Here's how the part is built. I have some questions about the finished solid (model axes, mm). Round coordinates to 2 decimals unless told otherwise and drop trailing zeros. Loops run counter-clockwise (first coordinate to the right, second up) from the corner with the lowest first, then second, coordinate; pieces in that order, holes last. Notation, with made-up numbers: M 46,22.5 L 58,22.5 A17 cw 58,50.5 Z; hole C 79.25,-19.75 d8. An arc over 180 degrees is marked long. Answer as CSV lines item,"result".
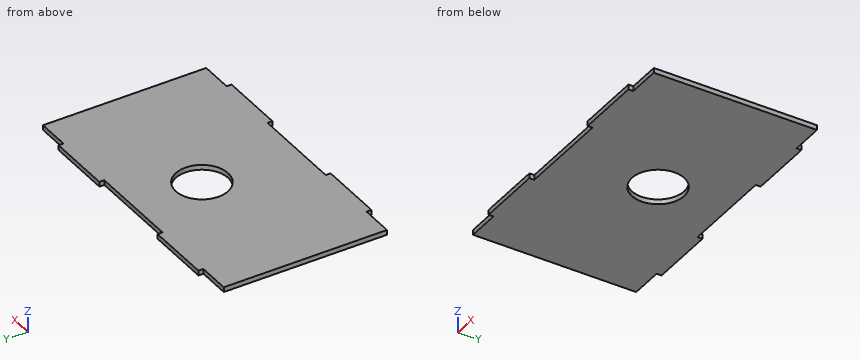
```python
from build123d import *

# Parameters (mm, degrees)
SKETCH1_R           = 16
BOSS_EXTRUDE1_DEPTH = 1.5


with BuildPart() as part:
    # Sketch1 → Boss-Extrude1 (new body, symmetric)
    with BuildSketch(Plane.XY):
        Polygon((-28.5, 50), (28.5, 50), (28.5, 53), (68.5, 53), (68.5, 50), (88.5, 50), (88.5, -50), (68.5, -50), (68.5, -53), (28.5, -53), (28.5, -50), (-28.5, -50), (-28.5, -53), (-68.5, -53), (-68.5, -50), (-88.5, -50), (-88.5, 50), (-68.5, 50), (-68.5, 53), (-28.5, 53), align=None)
        with Locations((0, 8)):
            Circle(SKETCH1_R, mode=Mode.SUBTRACT)
    extrude(amount=BOSS_EXTRUDE1_DEPTH, both=True)


solid = part.part
```
1. I want a section at D-D, the plane x = -76. Please give me the cut outline in (y, z), and give its area (3 significant figures).
Evaluation:
outline,"M -50,-1.5 L 50,-1.5 L 50,1.5 L -50,1.5 Z"
area,"300 mm²"
2. I want a section at B-B, the plane y = 8. Please give me the cut outline in (x, z), and give its area (3 significant figures).
Evaluation:
outline,"M -88.5,-1.5 L -16,-1.5 L -16,1.5 L -88.5,1.5 Z; M 16,-1.5 L 88.5,-1.5 L 88.5,1.5 L 16,1.5 Z"
area,"435 mm²"
3. I want a section at C-C, the plane z = -0.2. Please give me the cut outline in (x, y), and give its area (3 significant figures).
Evaluation:
outline,"M -88.5,-50 L -68.5,-50 L -68.5,-53 L -28.5,-53 L -28.5,-50 L 28.5,-50 L 28.5,-53 L 68.5,-53 L 68.5,-50 L 88.5,-50 L 88.5,50 L 68.5,50 L 68.5,53 L 28.5,53 L 28.5,50 L -28.5,50 L -28.5,53 L -68.5,53 L -68.5,50 L -88.5,50 Z; hole C 0,8 d32"
area,"17,400 mm²"
4. I want a section at A-A, the plane x = 0. Please give me the cut outline in (y, z).
Evaluation:
outline,"M -50,-1.5 L -8,-1.5 L -8,1.5 L -50,1.5 Z; M 24,-1.5 L 50,-1.5 L 50,1.5 L 24,1.5 Z"
5. If I drill on line 1 (Y direction, x = 0, z = -0.6); line 2 (X direction, y = 7.5, z = -1.2); line 3 (Y direction, x = -18, z = 0.7), over which ranges is the centre line in solid material (lowest first)? Write a range as [from, to].
Evaluation:
line 1,"y = [-50, -8], [24, 50]"
line 2,"x = [-88.5, -15.99], [15.99, 88.5]"
line 3,"y = [-50, 50]"
6. For P1, Ø0.9, axis at x = 83, z = 0, coming from the -Y side; P2, Ø19, axis at x = 0, y = 8, coming from the +Z side; P3, Ø1.5, axis at x = 83, z = 0, coming from the +Y side; P4, Ø1.5, axis at y = 51.5, z = 0.5, coming from the +X side, each with a flat end and sliding along its axis, tell me the tip position at first contact or that it passes through.
Evaluation:
P1,"stops at y = -50"
P2,"passes through"
P3,"stops at y = 50"
P4,"stops at x = 68.5"
